Geometry: final body of the model. Coordinates: model frame, mm. Face numbers are marked on the shaded views. A direction names the side the tool comes from. Give positions to 0.01 mm unless a question says otherwise; leave off trailing zeros. Order: outer loops, then holes, each group sorted by start corner. A loop starts at its lowest first (then second) coordinate and runs counter-clockwise, first axis right, second up. Notation, with made-up numbers: (24.5, 87.5) -> (77.5, 87.5) arc R16 ccw to (77.5, 94.5) -> close; hole circle Ø2 at (67, -39). An arc over 180 degrees is marked (long way). One line per question, with ' | ' between items. Start each with the question number.
(1) Mould query, pull axis Z, two halves, no side actions, for the marked faces 1, 2, 3 and 4. Classes: +Z half, -Z half, draft (parallel to the pull), parting line (faces both ways), or undercut.
(2) Section B-B (y = 0). Return loops of the section in (x, z).
(3) Section D-D (z = 57.5). Return loops of the section in (x, y), then the cut area to 3 significant figures.
(4) Set-up query: the marked faces 5, 6, 7 and 8. Return all of +Z, -Z, +X, -X, +Y, -Y with unobstructed straight access to the full face (end or side cutting, diameter ignored); none if empty.
(5) Section A-A (x = 0). Return loops of the section in (y, z).
(6) First-contact query: pin 1 Ø4 at (y, z) = (5, 16.5) entering from +X; pin 2 Ø3 at (x, y) = (6, 0) entering from +Z; pin 3 Ø9 at (x, z) = (0.5, 2) entering from +Y; pin 4 Ø6 at (x, z) = (1, 61) entering from +Y. Flat tips, straight axial feed; report the tip coordinate or a pass-through.
(7) Ray query, L1, parallel to X at y = -0.5, z = 66; L2, parallel to Z at x = 0, y = 2; L3, parallel to X at y = -0.25, z = 20.5. Return the intervals inside material, ascending.
(8) Section C-C (x = -5). Return loops of the section in (y, z).
```python
from build123d import *

# Parameters (mm, degrees)
F0_W           = 12.7
F0_H           = 80
F3_DEPTH       = 12.701
F3_DEPTH_BACK  = 12.701
F4_R           = 4
F5_DEPTH       = 11
F6_R           = 2
F7_DEPTH       = 10
F8_R           = 4
F9_R           = 1.55
F10_DEPTH      = 12.701
F10_DEPTH_BACK = 12.701


with BuildPart() as f1:
    # F0 (on Front) → F1 (revolve)
    with BuildSketch(Plane.XZ):
        with Locations((-6.35, 30)):
            Rectangle(F0_W, F0_H)
    revolve(axis=Axis((0, 0, 30), (0, 0, -1)))

    # F2 (on Right) → F3 (cut, two sides)
    with BuildSketch(Plane.YZ) as f3_sk:
        Polygon((-4, -10), (-4, 42), (-29.7404956073, 42), (-29.7404956073, -22.2334191203), (-4, -22.2334191203), align=None)
        Polygon((40.2332246304, 42), (4, 42), (4, -10), (4, -16.8698504567), (40.2332246304, -16.8698504567), align=None)
    extrude(amount=-F3_DEPTH, mode=Mode.SUBTRACT)
    extrude(f3_sk.sketch, amount=F3_DEPTH_BACK, mode=Mode.SUBTRACT)

    # F4 (on Front) → F5 (join, symmetric)
    with BuildSketch(Plane.XZ):
        Circle(F4_R)
    extrude(amount=F5_DEPTH, both=True)

    # F6 (on face) → F7 (cut)
    with BuildSketch(Plane.XY.offset(70)):
        with Locations((-6, 0)):
            Circle(F6_R)
        with Locations((6, 0)):
            Circle(F6_R)
    extrude(amount=-F7_DEPTH, mode=Mode.SUBTRACT)

    # F8
    f8_edges = [f1.edges().sort_by_distance(p)[0] for p in [
        (12.7, 0, -10),
        (-12.537366, -2.025944, -10),
        (-12.537366, 2.025944, -10),
    ]]
    fillet(f8_edges, radius=F8_R)

    # F9 (on Front) → F10 (cut, two sides)
    with BuildSketch(Plane.XZ) as f10_sk:
        with Locations((0, 55)):
            Circle(F9_R)
    extrude(amount=F10_DEPTH, mode=Mode.SUBTRACT)
    extrude(f10_sk.sketch, amount=-F10_DEPTH_BACK, mode=Mode.SUBTRACT)


solid = f1.part
```
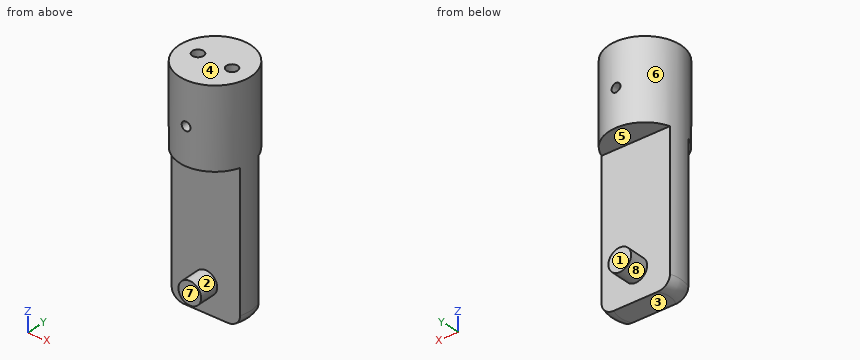
Response:
1) face 1: draft | face 2: undercut | face 3: -Z half | face 4: +Z half
2) outline: (-12.7, -6) arc R4 ccw to (-8.7, -10) -> (8.7, -10) arc R4 ccw to (12.7, -6) -> (12.7, 70) -> (8, 70) -> (8, 60) -> (4, 60) -> (4, 70) -> (-4, 70) -> (-4, 60) -> (-8, 60) -> (-8, 70) -> (-12.7, 70) -> close; hole circle Ø3.1 at (0, 55)
3) outline: circle Ø25.4 at (0, 0) | area: 507 mm^2
4) face 5: +X, -X, +Y | face 6: +Z, -Z | face 7: -Z, +X, -X, -Y | face 8: +Y
5) outline: (-12.7, 42) -> (-4, 42) -> (-4, 4) -> (-11, 4) -> (-11, -4) -> (-4, -4) -> (-4, -10) -> (4, -10) -> (4, -4) -> (11, -4) -> (11, 4) -> (4, 4) -> (4, 42) -> (12.7, 42) -> (12.7, 53.45) -> (-12.7, 53.45) -> close; (-12.7, 56.55) -> (12.7, 56.55) -> (12.7, 70) -> (-12.7, 70) -> close
6) pin 1: stops at x = 12.34 | pin 2: stops at z = 60 | pin 3: stops at y = 11 | pin 4: stops at y = 12.7
7) L1: x = -12.69 to -7.94, -4.06 to 4.06, 7.94 to 12.69 | L2: z = -10 to 53.45, 56.55 to 70 | L3: x = -12.7 to 12.7
8) outline: (-11.67, 42) -> (-4, 42) -> (-4, -10) -> (4, -10) -> (4, 42) -> (11.67, 42) -> (11.67, 70) -> (1.73, 70) -> (1.73, 60) -> (-1.73, 60) -> (-1.73, 70) -> (-11.67, 70) -> close
